Design review of the part built by this model. Coordinates are the model's own, in mm. A direction names the side the tool comes from. Coordinates: 2 decimals unless noted, no trailing zeros. Loops run counter-clockwise (first coordinate to the right, second up) from the corner with the lowest first, then second, coordinate; pieces in that order, holes last. Notation, with made-up numbers: (15.5, 69) - (35.5, 69) arc R20 ccw to (35.5, 104) - close; hole circle Ø9 at (23.25, -16.75). An arc over 180 degrees is marked (long way). One line per question, with ' | ' between items.
from build123d import *

# Parameters (mm, degrees)
SKETCH1_R           = 4.75
BOSS_EXTRUDE1_DEPTH = 30
SKETCH2_W           = 2.3
SKETCH2_H           = 6.8
CUT_EXTRUDE1_DEPTH  = 30
BOSS_EXTRUDE2_DEPTH = 3


with BuildPart() as part:
    # Sketch1 → Boss-Extrude1 (new body)
    with BuildSketch(Plane(origin=(0, 0, 0), x_dir=(0, 0, -1), z_dir=(1, 0, 0))):
        Circle(SKETCH1_R)
    extrude(amount=BOSS_EXTRUDE1_DEPTH)

    # Sketch2 → Cut-Extrude1 (cut)
    with BuildSketch(Plane(origin=(30, 0, 0), x_dir=(0, 0, -1), z_dir=(1, 0, 0))):
        Rectangle(SKETCH2_W, SKETCH2_H)
    extrude(amount=-CUT_EXTRUDE1_DEPTH, mode=Mode.SUBTRACT)

    # Sketch3 → Boss-Extrude2 (add)
    with BuildSketch(Plane.ZY):
        Polygon((5.773502692, 0), (2.886751346, 5), (-2.886751346, 5), (-5.773502692, 0), (-2.886751346, -5), (2.886751346, -5), align=None)
    extrude(amount=-BOSS_EXTRUDE2_DEPTH)


solid = part.part
Q1. To check wall thickness, follow line 1 along Y through (x, z) = (10, 0); line 2 along Z through (x, y) = (14.5, -0.25); line 3 along Z through (x, y) = (16, 1.25). State the ranges of each line that lie inside material, in increasing order.
Returned:
line 1: y = -4.75 to -3.4, 3.4 to 4.75 | line 2: z = -4.74 to -1.15, 1.15 to 4.74 | line 3: z = -4.58 to -1.15, 1.15 to 4.58
Q2. Take a section at C-C (y = 1.5). Give the boundary of the cut face in (x, z), plus the area to 3 significant figures.
Returned:
outline: (0, -4.91) - (3, -4.91) - (3, -4.51) - (30, -4.51) - (30, -1.15) - (3, -1.15) - (3, 1.15) - (30, 1.15) - (30, 4.51) - (3, 4.51) - (3, 4.91) - (0, 4.91) - close | area: 211 mm²
Q3. Draft analysis for pull direction Y (two halves, no side actions). For faces 1 (the flat face through (17, -3.4, 0)), 2 (the flat face through (0, 0, 0)), 3 (the flat face through (1.479, 2.465, 4.35)), state which applies: +Y half, -Y half, draft (parallel to the pull), parting line (faces both ways), or undercut.
Returned:
face 1: undercut | face 2: draft | face 3: +Y half
Q4. Take a section at A-A (x = 18.25). Give the boundary of the cut face in (y, z), plus the area to 3 significant figures.
Returned:
outline: circle Ø9.5 at (0, 0); hole (-3.4, -1.15) - (3.4, -1.15) - (3.4, 1.15) - (-3.4, 1.15) - close | area: 55.2 mm²
Q5. Tool access review of faces 4 (the flat face through (17, 3.4, 0)), 5 (the flat face through (1, -5, 0)): name each direction out of +Z, -Z, +X, -X, +Y, -Y from which nothing blocks a thin tool from reaching the whole face with its end or side.
Returned:
face 4: +X | face 5: +Z, -Z, +X, -X, -Y
Q6. Take a section at B-B (z = 0). Give the boundary of the cut face in (x, y).
Returned:
outline: (0, -5) - (3, -5) - (3, -4.75) - (30, -4.75) - (30, -3.4) - (3, -3.4) - (3, 3.4) - (30, 3.4) - (30, 4.75) - (3, 4.75) - (3, 5) - (0, 5) - close
Q7. For pin 1 (2 mm diameter, centred on x = 12, y = -1.5, fed in from +Z); pin 2 (2.5 mm diameter, centred on y = -0.5, z = -0.5, fed in from +X); pin 3 (1.2 mm diameter, centred on x = 23, z = 0, fed in from -Y); pin 4 (1.2 mm diameter, centred on x = 22.5, z = 0.5, fed in from +Y), all flat-tipped, find the tip position at first contact; note any pin that passes through.
Returned:
pin 1: stops at z = 4.72 | pin 2: stops at x = 30 | pin 3: stops at y = -4.75 | pin 4: stops at y = 4.75
Q8. Take a section at D-D (z = -2). Give the boundary of the cut face in (x, y).
Returned:
outline: (0, -5) - (3, -5) - (3, -4.31) - (30, -4.31) - (30, 4.31) - (3, 4.31) - (3, 5) - (0, 5) - close
